from build123d import *

# Parameters (mm, degrees)
F2_SIZE = 6


with BuildPart() as f1:
    # F0 (on Right) → F1 (revolve)
    with BuildSketch(Plane.YZ):
        Polygon((15, 6), (35, 6), (35, 17.5), (0, 17.5), (0, 15), (15, 15), align=None)
    revolve(axis=Axis((0, 7.5, 0), (0, 1, 0)))

    # F2
    f2_edges = [f1.edges().sort_by_distance(p)[0] for p in [
        (0, 35, -17.5),
    ]]
    chamfer(f2_edges, length=F2_SIZE)


solid = f1.part
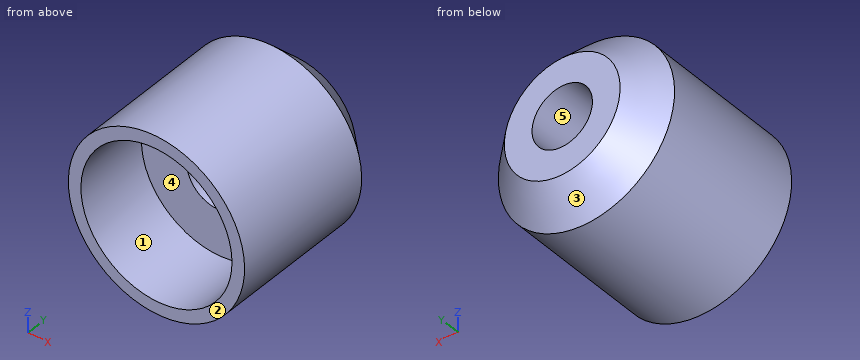
Design review of the part built by this model. Coordinates are the model's own, in mm. Face numbers are marked on the shaded views. A direction names the side the tool comes from. Give positions to 0.01 mm unless a question says otherwise; leave off trailing zeros. Loops run counter-clockwise (first coordinate to the right, second up) from the corner with the lowest first, then second, coordinate; pieces in that order, holes last. Notation, with made-up numbers: M -2.75,71 L 22.25,71 A24 ccw 22.25,101 Z; hole C -27,-9.5 d6. An arc over 180 degrees is marked long. Answer as a JSON object with one key per item and string values.
Item 1: For P1, Ø12, axis at x = 9, y = 4, coming from the +Z side; P2, Ø1.5, axis at x = 13.5, z = -0.5, coming from the -Y side; P3, Ø1.5, axis at x = 13, y = 17, coming from the -Z side, all flat-tipped, find the tip position at first contact; note any pin that passes through.
Output values:
{"P1": "stops at z = 17.24", "P2": "stops at y = 15", "P3": "stops at z = -12.5"}
Item 2: We need section B-B (z = 0). State the section outline as (x, y) points, and give its area (3 significant figures).
Output values:
{"outline": "M -17.5,0 L -15,0 L -15,15 L -6,15 L -6,35 L -11.5,35 L -17.5,29 Z; M 6,15 L 15,15 L 15,0 L 17.5,0 L 17.5,29 L 11.5,35 L 6,35 Z", "area": "499 mm2"}
Item 3: We need section C-C (y = 21.5). State the section outline as (x, z) points.
Output values:
{"outline": "C 0,0 d35; hole C 0,0 d12"}
Item 4: We need section A-A (x = 0). State the section outline as (y, z) points.
Output values:
{"outline": "M 0,-17.5 L 29,-17.5 L 35,-11.5 L 35,-6 L 15,-6 L 15,-15 L 0,-15 Z; M 0,15 L 15,15 L 15,6 L 35,6 L 35,11.5 L 29,17.5 L 0,17.5 Z"}
Item 5: Machinability: for the marked faces 4 and 5, which of the approach directions +Z, -Z, +X, -X, +Y, -Y give a long, thin tool a straight path to every point of the face, cutting with its end or side? Answer none if there is none.
Output values:
{"face 4": "-Y", "face 5": "+Y, -Y"}
Item 6: We need section D-D (y = 9.5). State the section outline as (x, z) points, and give its area (3 significant figures).
Output values:
{"outline": "C 0,0 d35; hole C 0,0 d30", "area": "255 mm2"}
Item 7: Wall thickness on line 1 along X through (y, z) = (26, 0); line 2 along X through (y, z) = (3.75, 0); line 3 along Y through (x, z) = (-7.5, -8.5): over which ranges is each line inside the solid? List them lowest first.
Output values:
{"line 1": "x = -17.5 to -6, 6 to 17.5", "line 2": "x = -17.5 to -15, 15 to 17.5", "line 3": "y = 15 to 35"}
Item 8: Mouldability with a two-part tool opening along Z and no side actions: class the marked faces 1, 2 and 3 as pulls with the +Z half, pulls with the -Z half, needs draft (parallel to the pull), parting line crosses it, or undercut.
Output values:
{"face 1": "undercut", "face 2": "needs draft", "face 3": "parting line crosses it"}
